Part model, mm, in its own coordinate system. A direction names the side the tool comes from. Coordinates: 2 decimals unless noted, no trailing zeros. Loops run counter-clockwise (first coordinate to the right, second up) from the corner with the lowest first, then second, coordinate; pieces in that order, holes last. Notation, with made-up numbers: M -2.75,78 L 46.25,78 A23 cw 46.25,94 Z; hole C 76,35 d8. An arc over 180 degrees is marked long. Use a Markdown table: item, result. Add a question column.
1) Pin check, flat tips, straight feed: pin 1 Ø7 at (x, y) = (224, -2.5) entering from -Z; pin 2 Ø6.5 at (x, y) = (-226, 0) entering from +Z; pin 3 Ø4 at (x, y) = (42, -8.5) entering from -Z; pin 4 Ø8.5 at (x, y) = (-226, 0) entering from +Z. Stop position of each tip, or through.
2) Pull direction X, two halves, no side cores. Call faces 4 (the flat face through (-3, 12, 24)), 5 (the flat face through (250, 0, 24)), 6 (the flat face through (-229, -3, 12)): released by +X, released by -X, zero draft, split by the parting line, or undercut.
3) Band-saw the part on A-A (z = 6.5). List the corners of the cut face in (x, y), plus the area to 3 significant figures.
4) Band-saw the part on B-B (y = 0). State how many separate pieces and enclosed holes the cut face has, plus the area to 3 significant figures.
5) Tool access for faces 1 (the cylindrical face through (222, 0, 24)), 2 (the flat face through (-226.1, -4.3, 36)), 3 (the cylindrical face through (-232.466, -2.681, 5.916)): list every direction of +Z, -Z, +X, -X, +Y, -Y with a clear straight run to the whole face (end or side of a thin tool).
6) Wall check: probe 1 along Y at (x, z) = (-226, 41); probe 2 along Y at (x, z) = (0, 9.5); probe 3 along X at (y, z) = (-6, 44.5). Give the ranges that are in metal, low to high. Write a range as from..to.
from build123d import *

# Parameters (mm, degrees)
ESQUISSE1_W             = 500
ESQUISSE1_H             = 24
BOSS_EXTRU_1_DEPTH      = 48
ESQUISSE2_R             = 4
ENL_V_MAT_EXTRU_1_DEPTH = 255.848974885
ESQUISSE3_R             = 10
ENL_V_MAT_EXTRU_2_DEPTH = 12
ESQUISSE4_R             = 7
ENL_V_MAT_EXTRU_3_DEPTH = 12


with BuildPart() as part:
    # Esquisse1 → Boss.-Extru.1 (new body)
    with BuildSketch(Plane.XY):
        Rectangle(ESQUISSE1_W, ESQUISSE1_H)
    extrude(amount=BOSS_EXTRU_1_DEPTH)

    # Esquisse2 → Enlèv. mat.-Extru.1 (cut, through all)
    with BuildSketch(Plane.XY.offset(48)):
        with Locations((-226, 0)):
            Circle(ESQUISSE2_R)
        Circle(ESQUISSE2_R)
        with Locations((226, 0)):
            Circle(ESQUISSE2_R)
    extrude(amount=-ENL_V_MAT_EXTRU_1_DEPTH, mode=Mode.SUBTRACT)

    # Esquisse3 → Enlèv. mat.-Extru.2 (cut)
    with BuildSketch(Plane.XY.offset(48)):
        with Locations((-226, 0)):
            Circle(ESQUISSE3_R)
        Circle(ESQUISSE3_R)
        with Locations((226, 0)):
            Circle(ESQUISSE3_R)
    extrude(amount=-ENL_V_MAT_EXTRU_2_DEPTH, mode=Mode.SUBTRACT)

    # Esquisse4 → Enlèv. mat.-Extru.3 (cut)
    with BuildSketch(Plane(origin=(0, 0, 0), x_dir=(-1, 0, 0), z_dir=(0, 0, -1))):
        with Locations((-226, 0)):
            Circle(ESQUISSE4_R)
        Circle(ESQUISSE4_R)
        with Locations((226, 0)):
            Circle(ESQUISSE4_R)
    extrude(amount=-ENL_V_MAT_EXTRU_3_DEPTH, mode=Mode.SUBTRACT)


solid = part.part
Entries:
| question | item | result |
|---|---|---|
| 1 | pin 1 | z = 12 |
| 1 | pin 2 | through |
| 1 | pin 3 | z = 0 |
| 1 | pin 4 | z = 36 |
| 2 | face 4 | zero draft |
| 2 | face 5 | released by +X |
| 2 | face 6 | undercut |
| 3 | outline | M -250,-12 L 250,-12 L 250,12 L -250,12 Z; hole C -226,0 d14; hole C 0,0 d14; hole C 226,0 d14 |
| 3 | area | 11,500 mm2 |
| 4 | separate pieces | 4 |
| 4 | enclosed holes | 0 |
| 4 | area | 22,200 mm2 |
| 5 | face 1 | +Z, -Z |
| 5 | face 2 | +Z |
| 5 | face 3 | -Z |
| 6 | probe 1 | -12..-10, 10..12 |
| 6 | probe 2 | -12..-7, 7..12 |
| 6 | probe 3 | -250..-234, -218..-8, 8..218, 234..250 |
